Read the model definition and answer for the solid it produces. Units are mm, in the model's axes. Face numbers are marked on the shaded views. Coordinates: 2 decimals unless noted, no trailing zeros. Loops run counter-clockwise (first coordinate to the right, second up) from the corner with the lowest first, then second, coordinate; pieces in that order, holes last. Notation, with made-up numbers: (-14.75, 80) - (1.25, 80) arc R25 ccw to (1.25, 107) - close; hole circle Ø2 at (20.5, 27.25). An arc over 180 degrees is marked (long way). Use CSV: the item, a comma, the result in double quotes.
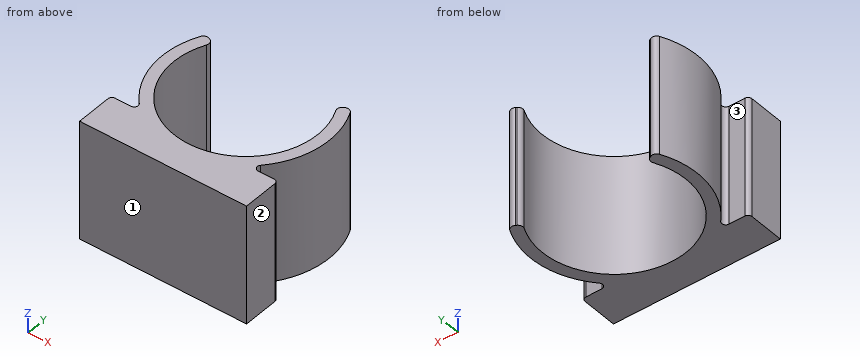
```python
from build123d import *

# Parameters (mm, degrees)
PAD001_DEPTH = 30
FILLET_R     = 1.3
FILLET001_R  = 1


with BuildPart() as part:
    # Sketch001 → Pad001 (new body)
    with BuildSketch(Plane.XY):
        with BuildLine():
            ThreePointArc((-18.186533, 28.6), (-20.679194, 14.443373), (-13.482952, 2))
            Line((-21, 2), (-13.482952, 2))
            Line((-21, -7.9), (-21, 2))
            Line((21, -7.9), (-21, -7.9))
            Line((21, 2), (21, -7.9))
            Line((13.482952, 2), (21, 2))
            ThreePointArc((13.482952, 2), (20.679194, 14.443373), (18.186533, 28.6))
            Line((18.186533, 28.6), (15.67506, 27.15))
            ThreePointArc((-15.67506, 27.15), (0, 0), (15.67506, 27.15))
            Line((-18.186533, 28.6), (-15.67506, 27.15))
        make_face()
    extrude(amount=PAD001_DEPTH)

    # Fillet
    fillet_edges = [part.edges().sort_by_distance(p)[0] for p in [
        (-15.67506, 27.15, 15),
        (-18.186533, 28.6, 15),
        (15.67506, 27.15, 15),
        (18.186533, 28.6, 15),
    ]]
    fillet(fillet_edges, radius=FILLET_R)

    # Fillet001
    fillet001_edges = [part.edges().sort_by_distance(p)[0] for p in [
        (-13.482952, 2, 15),
        (13.482952, 2, 15),
        (21, 2, 15),
        (-21, 2, 15),
    ]]
    fillet(fillet001_edges, radius=FILLET001_R)


solid = part.part
```
Q1. Find the intervals of material crossed by probe 1 along X at (y, z) = (18.1, 24); probe 2 along Y at (x, z) = (0, 22.5); probe 3 along X at (y, z) = (8.5, 26.25), in increasing order. Write a range as [from, to].
Reported:
probe 1,"x = [-21, -18.1], [18.1, 21]"
probe 2,"y = [-7.9, 0]"
probe 3,"x = [-18.68, -15.34], [15.34, 18.68]"
Q2. Given P1, Ø2, axis at x = 19, z = 10, coming from the +Y side; P2, Ø21.5, axis at x = 0, y = 18.1, coming from the -Z side, each flat-ended and moving along its own axis, determine where each tip first touches the part or whether it passes through.
Reported:
P1,"stops at y = 28.06"
P2,"passes through"
Q3. The part is cut by section C-C on y = 7. Determine the outline of the cut face in (x, z), and give its area (3 significant figures).
Reported:
outline,"(-17.83, 0) - (-14.3, 0) - (-14.3, 30) - (-17.83, 30) - close; (14.3, 0) - (17.83, 0) - (17.83, 30) - (14.3, 30) - close"
area,"212 mm²"
Q4. The part is cut by section D-D on x = 0. Determine the outline of the cut face in (y, z), and give its area (3 significant figures).
Reported:
outline,"(-7.9, 0) - (0, 0) - (0, 30) - (-7.9, 30) - close"
area,"237 mm²"
Q5. For a pull along Y with two mould halves and no side action, classify the marked faces 1, 2 and 3 as +Y half, -Y half, draft (parallel to the pull), parting line (faces both ways), or undercut.
Reported:
face 1,"-Y half"
face 2,"draft"
face 3,"undercut"
Q6. The part is cut by section B-B on z = 26.25. Determine the outline of the cut face in (x, y).
Reported:
outline,"(-21, -7.9) - (21, -7.9) - (21, 1) arc R1 ccw to (20, 2) - (16, 2) arc R1 cw to (15.27, 3.69) arc R21 ccw to (18.84, 27.38) arc R1.3 ccw to (17.02, 27.93) - (16.76, 27.78) arc R1.3 ccw to (16.25, 26.08) arc R18.1 cw (long way) to (-16.25, 26.08) arc R1.3 ccw to (-16.76, 27.78) - (-17.02, 27.93) arc R1.3 ccw to (-18.84, 27.38) arc R21 ccw to (-15.27, 3.69) arc R1 cw to (-16, 2) - (-20, 2) arc R1 ccw to (-21, 1) - close"
Q7. The part is cut by section A-A on y = 18.1. Determine the outline of the cut face in (x, z).
Reported:
outline,"(-21, 0) - (-18.1, 0) - (-18.1, 30) - (-21, 30) - close; (18.1, 0) - (21, 0) - (21, 30) - (18.1, 30) - close"
